Could you check a few things on this model? Use its own coordinates, in mm. Give positions to 0.01 mm unless a question says otherwise; leave off trailing zeros. Loops run counter-clockwise (first coordinate to the right, second up) from the corner with the lowest first, then second, coordinate; pieces in that order, holes last. Notation, with made-up numbers: (-21, -30) - (20, -30) arc R22 cw to (20, -10) - close; hole circle Ø8 at (59, 29.5). An arc over 180 degrees is marked (long way). Use CSV: the item, a comma, the result in double quotes.
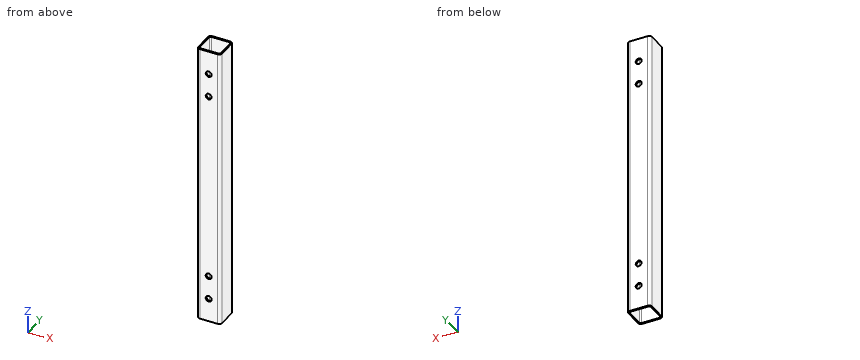
from build123d import *

# Parameters (mm, degrees)
SKETCH1_W          = 25.4
SKETCH1_H          = 25.4
BASE_EXTRUDE_DEPTH = 152.4
FILLET1_R          = 3.175
SHELL1_T           = -1.5875
SKETCH5_R          = 3.175
CUT_EXTRUDE2_DEPTH = 156.02325632


with BuildPart() as part:
    # Sketch1 → Base-Extrude (new, symmetric)
    with BuildSketch(Plane.XY):
        Rectangle(SKETCH1_W, SKETCH1_H)
    extrude(amount=BASE_EXTRUDE_DEPTH, both=True)

    # Fillet1
    fillet1_edges = [part.edges().sort_by_distance(p)[0] for p in [
        (-12.7, 12.7, 0),
        (12.7, 12.7, 0),
        (12.7, -12.7, 0),
        (-12.7, -12.7, 0),
    ]]
    fillet(fillet1_edges, radius=FILLET1_R)

    # Shell1
    shell1_openings = [part.faces().sort_by_distance(p)[0] for p in [
        (0, 0, 152.4),
        (0, 0, -152.4),
    ]]
    offset(amount=SHELL1_T, openings=shell1_openings, kind=Kind.INTERSECTION)

    # Sketch5 → Cut-Extrude2 (cut, through all)
    with BuildSketch(Plane.XZ.offset(12.7)):
        with Locations((0, 127)):
            Circle(SKETCH5_R)
        with Locations((0, 101.6)):
            Circle(SKETCH5_R)
        with Locations((0, -127)):
            Circle(SKETCH5_R)
        with Locations((0, -101.6)):
            Circle(SKETCH5_R)
    extrude(amount=-CUT_EXTRUDE2_DEPTH, mode=Mode.SUBTRACT)


solid = part.part
1) Suppose I cut it at B-B (x = 7). Please give me the cut outline in (y, z), plus the area to 3 significant figures.
Answer below:
outline,"(-12.7, -152.4) - (-11.11, -152.4) - (-11.11, 152.4) - (-12.7, 152.4) - close; (11.11, -152.4) - (12.7, -152.4) - (12.7, 152.4) - (11.11, 152.4) - close"
area,"968 mm2"
2) I need wall thicknesses on line 1 along Z through (x, y) = (0, 11.75) (3 decimals); line 2 along X through (y, z) = (-8, 97). Which ranges of each line are inside material? Lowest first, please.
Answer below:
line 1,"z = -152.4 to -130.175, -123.825 to -104.775, -98.425 to 98.425, 104.775 to 123.825, 130.175 to 152.4"
line 2,"x = -12.7 to -11.11, 11.11 to 12.7"
3) I'm going to push a flat-ended pin straight in: P1, Ø5, axis at x = 0, z = 127, coming from the -Y side. Where does the tip first touch, or does it pass through?
Answer below:
P1,"passes through"
